For this review, take the finished solid that the model builds, in its own axes (mm). Face numbers are marked on the shaded views. A direction names the side the tool comes from. Coordinates: 2 decimals unless noted, no trailing zeros. Loops run counter-clockwise (first coordinate to the right, second up) from the corner with the lowest first, then second, coordinate; pieces in that order, holes last. Notation, with made-up numbers: M 81.5,83 L 88.5,83 A16 cw 88.5,101 Z; hole C 57,15.5 d5. An arc over 180 degrees is marked long. Write each question's results on one line, items separated by ' | '. Start each with the question number.
```python
from build123d import *

# Parameters (mm, degrees)
F0_W   = 98
F0_H   = 5
F0_W_2 = 2
F0_H_2 = 7.5


with BuildPart() as f1:
    # F0 (on Top) → F1 (revolve)
    with BuildSketch(Plane.XY):
        with BuildLine():
            Line((0, 10), (0, 0))
            Line((0, 0), (80, 0))
            Line((80, 0), (80, 7.5))
            add(Edge.make_bspline(
                [(80, 7.5), (77.4320963341, 5.4602127374), (64.9277701604, 8.6077862709), (53.6662401112, 12.0157463446), (50.0245369175, 12.5048198747), (46.3291163152, 12.9393686412), (36.7743339747, 8.9436592945), (24.9276027824, 9.9274888653), (21.6319746465, 10.5063086165), (10.220435011, 5.9188095094), (4.6241535969, 8.6259927698), (0, 10)],
                knots=[0, 0, 0, 0, 0.1463849193, 0.2822756936, 0.3513645208, 0.4207173296, 0.544584059, 0.6744916377, 0.7457775925, 0.8705254251, 1, 1, 1, 1], degree=3))
        make_face()
        Polygon((-2, 0), (0, 0), (0, 10), (-2, 10), (-2, 5), align=None)
        with Locations((-51, 2.5)):
            Rectangle(F0_W, F0_H)
        with Locations((81, 3.75)):
            Rectangle(F0_W_2, F0_H_2)
    revolve(axis=Axis((-50, 0, 0), (-1, 0, 0)))


solid = f1.part
```
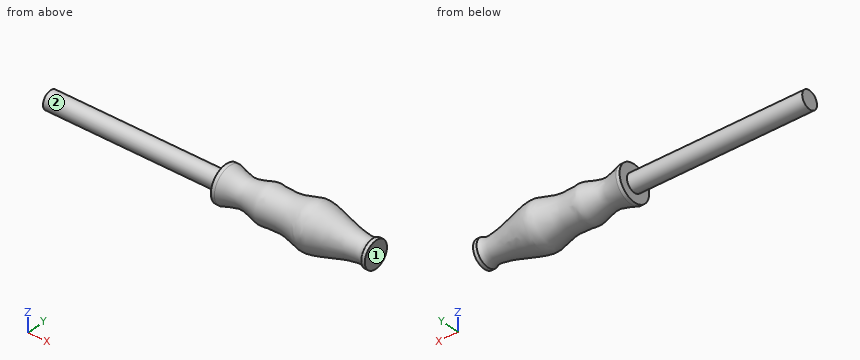
Q1. Insertion check: P1, Ø6, axis at y = -0.5, z = 8, coming from the +X side; P2, Ø1, axis at x = 16.5, z = 6.5, coming from the +Y side; P3, Ø2, axis at y = -9, z = 1, coming from the -X side; P4, Ø6, axis at x = 28.5, z = -0.5, coming from the +Y side. Each pin has a flat end and moves straight along its axis. Give the tip position at first contact, or say it passes through.
Q2. To check wall thickness, follow line 1 along Z through (x, y) = (-66.5, -0.75); line 2 along Y through (x, z) = (-9, -3); line 3 along Y through (x, z) = (45.5, 6). State the ranges of each line that lie inside material, in increasing order.
Q3. Take a section at A-A, the plane x = -36. Give the boundary of the cut face in (y, z), then the cut area to 3 significant figures.
Q4. For the marked faces 1 and 2, list the 3-axis set-ups (+Z, -Z, +X, -X, +Y, -Y) from which the entire face can be reached by the end or side of a thin tool; tool diameter is ignored.
Results:
1) P1: x = 82 | P2: y = 6.16 | P3: x = -2 | P4: y = 9.94
2) line 1: -4.94 to 4.94 | line 2: -4 to 4 | line 3: -10.66 to 10.66
3) outline: C 0,0 d10 | area: 78.5 mm^2
4) face 1: +Z, -Z, +X, +Y, -Y | face 2: -X
